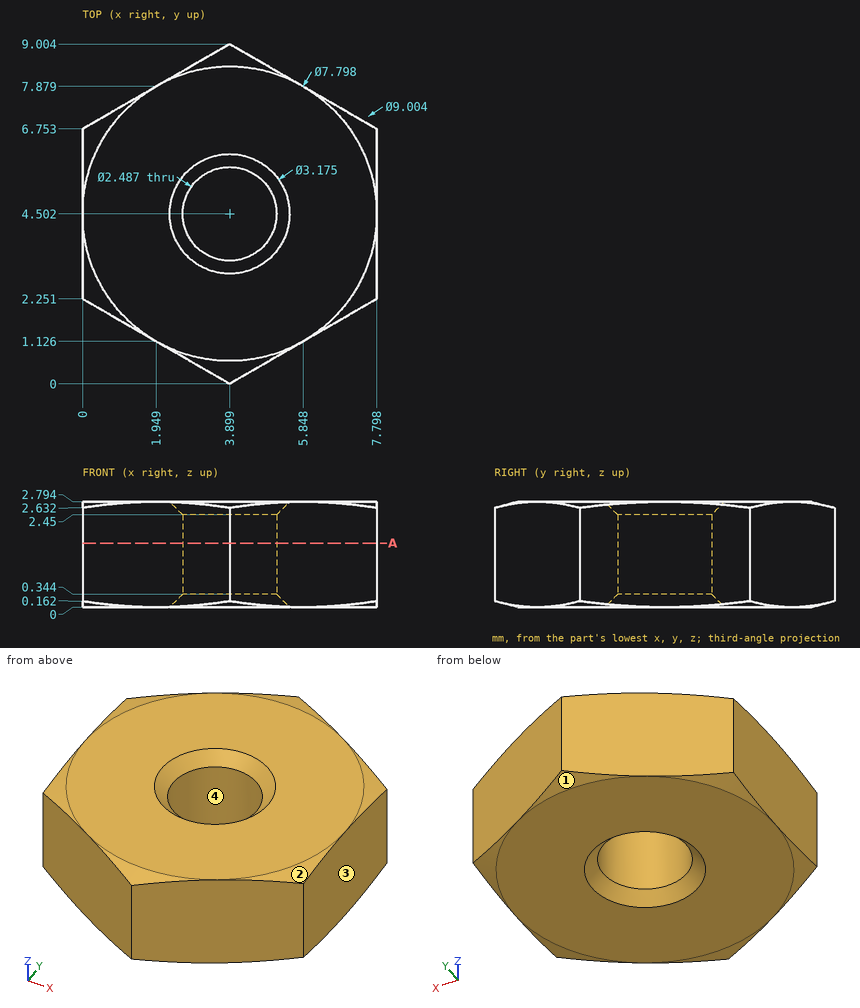
The figure shows three views and two pictorial views of one solid part (mm, origin at its lowest corner). Answer the questions. Give positions to 0.01 mm unless a question says otherwise; leave off trailing zeros. Order: outer loops, then holes, each group sorted by start corner. A loop starts at its lowest first (then second) coordinate and runs counter-clockwise, first axis right, second up. Notation, with made-up numbers: (47, -29.75) - (90, -29.75) arc R20 cw to (90, -3.75) - close; hole circle Ø11 at (-27, 55). An arc over 180 degrees is marked (long way). Answer as CSV lines item,"result".
Q1. Determine the mould class of the marked faces 1, 2, 3 and 4 for opening direction Y: pulls with the +Y half, pulls with the -Y half, needs draft (parallel to the pull), parting line crosses it, or undercut.
Answer key:
face 1,"pulls with the +Y half"
face 2,"pulls with the -Y half"
face 3,"needs draft"
face 4,"undercut"
Q2. Straight lines are drawn through the part: L1, parallel to Y at x = 4.75, z = 2.25 (1 decimal); L2, parallel to X at y = 3.5, z = 0.15 (1 decimal); L3, parallel to X at y = 4, z = 2 (1 decimal). For each, find the intervals that lie inside material, in ascending order.
Answer key:
L1,"y = 0.5 to 3.6, 5.4 to 8.5"
L2,"x = 0 to 2.9, 4.9 to 7.8"
L3,"x = 0 to 2.8, 5 to 7.8"
Q3. A cutting plane is placed at A-A, the plane z = 1.7. Determine the outline of the cut face in (x, y) (1 decimal).
Answer key:
outline,"(0, 2.3) - (3.9, 0) - (7.8, 2.3) - (7.8, 6.8) - (3.9, 9) - (0, 6.8) - close; hole circle Ø2.5 at (3.9, 4.5)"
Q4. This flat-tipped pin is pushed along its axis until it touches: pin 1 Ø1.5 at (x, z) = (6, 2) entering from -Y. Where does it stop, or does it pass through?
Answer key:
pin 1,"stops at y = 0.78"
